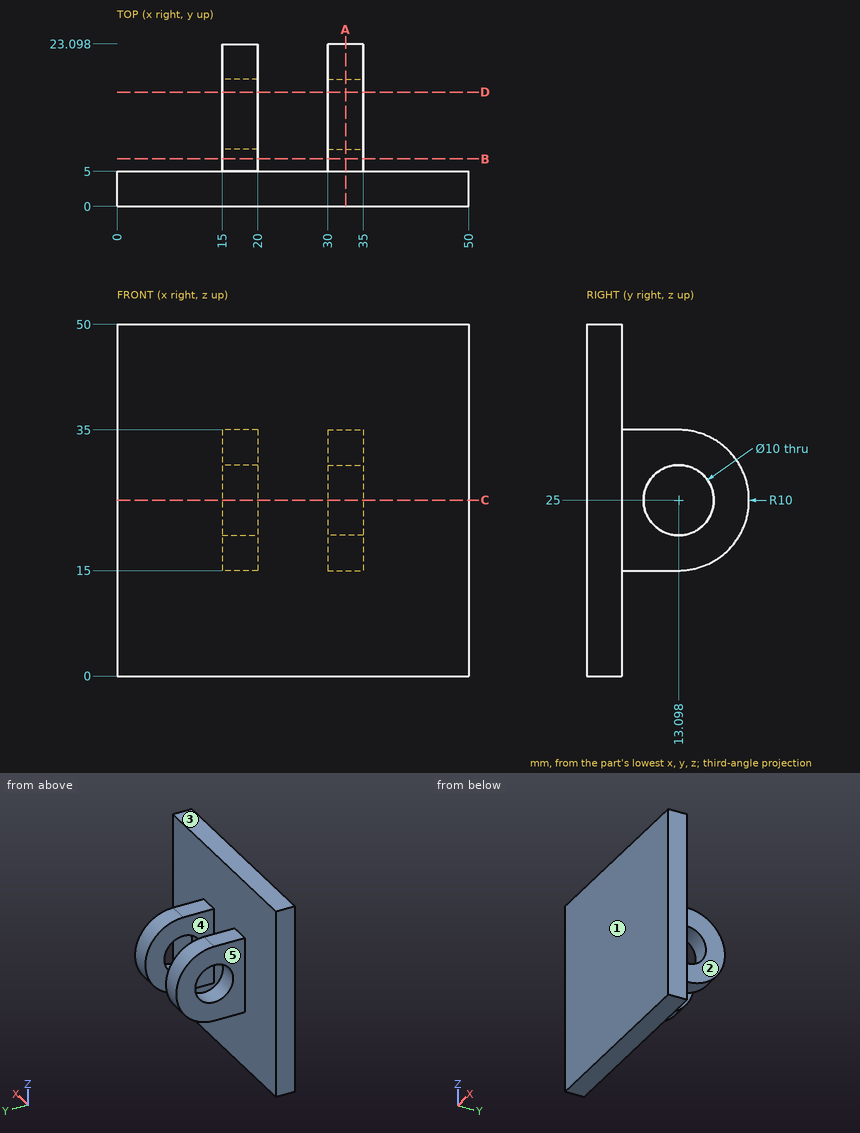
Drawing for the job (mm, zero at the part's lowest x, y, z). A direction names the side the tool comes from. Give positions to 0.01 mm unless a question says otherwise; leave off trailing zeros. Write each loop counter-clockwise with the first axis right and the second up, starting at its lowest first coordinate (ties: lowest second). Pieces come first, ordered by that corner, then holes. Notation, with made-up numbers: M -14.75,3.5 L 7.25,3.5 A18 ccw 7.25,28.5 Z; hole C 82,10 d7. An arc over 180 degrees is marked long. Return JSON: item names as keys, results as strings. Group by question number.
(1) Flat gauge pins, fed straight in: pin 1 Ø1.5 at (y, z) = (13, 31.5) entering from +X; pin 2 Ø12 at (x, y) = (24.5, 11.5) entering from +Z; pin 3 Ø1.5 at (x, y) = (18.5, 9) entering from -Z; pin 4 Ø25 at (x, z) = (25, 20.5) entering from +Y. Where does each tip first touch, or does it go through?
(2) 3-axis set-ups, long thin cutter, end or side, ignore diameter. For the marked faces 1 and 2: which of +Z, -Z, +X, -X, +Y, -Y reach the whole face in a straight line?
(3) Mould opens along X. For the marked faces 3, 4 and 5 say: pulls with the +X half, pulls with the -X half, needs draft (parallel to the pull), parting line crosses it, or undercut.
(4) Band-saw the part on A-A (x = 32.5). Give the cut face in (y, z).
(5) Drill centre lines: L1, parallel to Y at x = 32, z = 25; L2, parallel to X at y = 6.25, z = 27; L3, parallel to Y at x = 9.5, z = 25.5. Where is each one in solid material? Low to high. Write a range as [from, to].
(6) Band-saw the part on D-D (y = 16.25). Give the cut face in (x, z).
(7) Band-saw the part on B-B (y = 6.75). Give the cut face in (x, z), and give its area (3 significant figures).
(8) Band-saw the part on C-C (z = 25). Give the cut face in (x, y).
Entries:
{
 "1": {"pin 1": "stops at x = 35", "pin 2": "stops at z = 35", "pin 3": "stops at z = 15", "pin 4": "stops at y = 23.1"},
 "2": {"face 1": "+Z, -Z, +X, -X, -Y", "face 2": "+Z, -Z, +X, +Y"},
 "3": {"face 3": "needs draft", "face 4": "undercut", "face 5": "pulls with the -X half"},
 "4": {"outline": "M 0,0 L 5,0 L 5,15 L 13.1,15 A10 ccw 13.1,35 L 5,35 L 5,50 L 0,50 Z; hole C 13.1,25 d10"},
 "5": {"L1": "y = [0, 8.1], [18.1, 23.1]", "L2": "x = [15, 20], [30, 35]", "L3": "y = [0, 5]"},
 "6": {"outline": "M 15,15.51 L 20,15.51 L 20,21.12 L 15,21.12 Z; M 15,28.88 L 20,28.88 L 20,34.49 L 15,34.49 Z; M 30,15.51 L 35,15.51 L 35,21.12 L 30,21.12 Z; M 30,28.88 L 35,28.88 L 35,34.49 L 30,34.49 Z"},
 "7": {"outline": "M 15,15 L 20,15 L 20,35 L 15,35 Z; M 30,15 L 35,15 L 35,35 L 30,35 Z", "area": "200 mm^2"},
 "8": {"outline": "M 0,0 L 50,0 L 50,5 L 35,5 L 35,8.1 L 30,8.1 L 30,5 L 20,5 L 20,8.1 L 15,8.1 L 15,5 L 0,5 Z; M 15,18.1 L 20,18.1 L 20,23.1 L 15,23.1 Z; M 30,18.1 L 35,18.1 L 35,23.1 L 30,23.1 Z"}
}
